from build123d import *

# Parameters (mm, degrees)
F1_DEPTH = 8.636


with BuildPart() as f1:
    # F0 (on Front) → F1 (new body)
    with BuildSketch(Plane.XZ):
        with BuildLine():
            Line((-67.888543, 14.229136), (-67.888543, 8.327846))
            Line((-67.888543, 8.327846), (-67.590117, 5.694489))
            Line((-67.590117, 5.694489), (-10.072526, 2.980128))
            Line((-10.072526, 2.980128), (-3.732844, -4.12088))
            Line((-3.732844, -4.12088), (2.804628, -4.12088))
            Line((2.804628, -4.12088), (4.660426, -5.51241))
            Line((4.660426, -5.51241), (20.36539, -5.51241))
            ThreePointArc((20.36539, -5.51241), (22.326214, -6.957719), (24.524612, -8.006907))
            ThreePointArc((24.524612, -8.006907), (28.372895, -8.935837), (32.329973, -9.052986))
            ThreePointArc((32.329973, -9.052986), (35.941526, -8.275719), (38.847856, -5.995215))
            ThreePointArc((38.847856, -5.995215), (42.405349, -6.590703), (44.239189, -9.696728))
            Line((44.239189, -9.696728), (45.717698, -10.69943))
            ThreePointArc((45.717698, -10.69943), (45.850918, -13.592314), (47.728516, -15.797116))
            ThreePointArc((47.728516, -15.797116), (48.186683, -17.808436), (48.07616, -19.868318))
            ThreePointArc((48.07616, -19.868318), (47.693475, -23.337022), (49.28254, -26.443986))
            ThreePointArc((49.28254, -26.443986), (49.565033, -26.802415), (49.898703, -27.113765))
            Line((49.898703, -27.113765), (63.92391, -23.246003))
            Line((63.92391, -23.246003), (63.666757, -17.629698))
            Line((63.666757, -17.629698), (63.305743, -9.745057))
            ThreePointArc((63.305743, -9.745057), (62.05497, -4.640389), (59.587408, 0))
            ThreePointArc((59.587408, 0), (55.333048, 5.257953), (53.080335, 11.635331))
            Line((53.080335, 11.635331), (51.798906, 15.11586))
            Line((51.798906, 15.11586), (46.942841, 15.11586))
            ThreePointArc((46.942841, 15.11586), (46.45979, 13.035678), (45.55238, 11.102519))
            ThreePointArc((45.55238, 11.102519), (43.355932, 7.020729), (39.016269, 5.392008))
            Line((39.016269, 5.392008), (23.084078, 5.392008))
            Line((23.084078, 5.392008), (23.084078, 6.470653))
            Line((23.084078, 6.470653), (15.109499, 6.470653))
            Line((15.109499, 6.470653), (13.445796, 6.470653))
            Line((13.445796, 6.470653), (13.445796, 11.590629))
            Line((13.445796, 11.590629), (13.445796, 18.615682))
            Line((13.445796, 18.615682), (7.789209, 18.615682))
            Line((7.789209, 18.615682), (-7.699287, 18.537793))
            Line((-7.699287, 18.537793), (-4.879672, 18.475959))
            Line((-4.879672, 18.475959), (-4.879672, 14.229136))
            Line((-4.879672, 14.229136), (-7.699287, 14.229136))
            Line((-7.699287, 14.229136), (-67.888543, 14.229136))
        make_face()
        with BuildLine():
            ThreePointArc((18.888429, -1.232992), (20.03881, 1.476523), (22.555076, 3.004023))
            Line((22.555076, 3.004023), (28.890261, 3.004023))
            Line((28.890261, 3.004023), (32.984652, 3.004023))
            ThreePointArc((32.984652, 3.004023), (33.457255, 2.948329), (33.923268, 2.851961))
            ThreePointArc((33.923268, 2.851961), (37.989765, -1.51717), (35.673525, -7.018146))
            ThreePointArc((35.673525, -7.018146), (28.392646, -7.940351), (21.466842, -5.51241))
            Line((21.466842, -5.51241), (18.888429, -1.232992))
        make_face(mode=Mode.SUBTRACT)
        Polygon((-67.26525, 18.70371), (-67.888543, 14.229136), (-7.699287, 14.229136), (-7.699287, 18.537793), (-66.731323, 18.629336), align=None)
        Polygon((-65.611368, 15.894235), (-65.609761, 16.930796), (-61.958702, 16.97587), (-61.958702, 15.888571), align=None, mode=Mode.SUBTRACT)
        Polygon((-66.731323, 21.379774), (-66.731323, 18.629336), (-7.699287, 18.537793), (7.789209, 18.615682), (13.445796, 18.615682), (13.445796, 20.43255), (13.445796, 23.939529), (11.8609, 24.011148), (10.443351, 22.458594), (3.288107, 22.458594), (2.613084, 23.025269), (-3.514589, 23.025269), (-3.514589, 19.527677), (-59.21186, 19.614049), (-60.399957, 21.379774), align=None)
        Polygon((-66.20314, 22.302656), (-66.731323, 21.379774), (-60.399957, 21.379774), (-14.40332, 21.379774), (-13.479427, 23.025269), (-3.514589, 23.025269), (2.613084, 23.025269), (2.580326, 23.198023), (-17.181331, 23.198023), (-17.794525, 22.302656), align=None)
        with BuildLine():
            Line((-66.731323, 23.473777), (-66.20314, 22.302656))
            Line((-66.20314, 22.302656), (-17.794525, 22.302656))
            Line((-17.794525, 22.302656), (-17.181331, 23.198023))
            Line((-17.181331, 23.198023), (2.580326, 23.198023))
            Line((2.580326, 23.198023), (2.613084, 23.025269))
            Line((2.613084, 23.025269), (3.288107, 22.458594))
            Line((3.288107, 22.458594), (10.443351, 22.458594))
            Line((10.443351, 22.458594), (11.8609, 24.011148))
            Line((11.8609, 24.011148), (13.445796, 23.939529))
            Line((13.445796, 23.939529), (34.916848, 23.939529))
            Line((34.916848, 23.939529), (34.916848, 22.35744))
            Line((34.916848, 22.35744), (36.640268, 22.35744))
            Line((36.640268, 22.35744), (36.640268, 21.295426))
            Line((36.640268, 21.295426), (37.662946, 20.430082))
            Line((37.662946, 20.430082), (37.662946, 18.97577))
            Line((37.662946, 18.97577), (42.068332, 13.861337))
            Line((42.068332, 13.861337), (42.068332, 9.9928))
            Line((42.068332, 9.9928), (37.926942, 9.9928))
            Line((37.926942, 9.9928), (36.640268, 8.652356))
            Line((36.640268, 8.652356), (36.640268, 7.140663))
            Line((36.640268, 7.140663), (39.016269, 7.140663))
            ThreePointArc((39.016269, 7.140663), (40.885778, 7.338312), (42.642005, 8.008977))
            ThreePointArc((42.642005, 8.008977), (44.260743, 9.401881), (45.55238, 11.102519))
            ThreePointArc((45.55238, 11.102519), (46.45979, 13.035678), (46.942841, 15.11586))
            Line((46.942841, 15.11586), (51.798906, 15.11586))
            Line((51.798906, 15.11586), (51.798906, 16.040822))
            Line((51.798906, 16.040822), (45.381963, 19.682869))
            Line((45.381963, 19.682869), (42.202402, 18.006373))
            Line((42.202402, 18.006373), (40.930577, 18.006373))
            Line((40.930577, 18.006373), (38.329113, 19.682869))
            Line((38.329113, 19.682869), (38.329113, 25.174845))
            Line((38.329113, 25.174845), (38.329113, 28.956141))
            Line((38.329113, 28.956141), (16.867928, 28.956141))
            Line((16.867928, 28.956141), (15.879637, 29.998008))
            Line((15.879637, 29.998008), (15.187833, 29.998008))
            Line((15.187833, 29.998008), (11.387558, 29.998008))
            Line((11.387558, 29.998008), (5.248655, 27.211197))
            Line((5.248655, 27.211197), (-54.899268, 27.211197))
            Line((-54.899268, 27.211197), (-61.934408, 27.211197))
            Line((-61.934408, 27.211197), (-65.839738, 27.211197))
            Line((-65.839738, 27.211197), (-65.839738, 25.936976))
            Line((-65.839738, 25.936976), (-66.731323, 24.311243))
            Line((-66.731323, 24.311243), (-66.731323, 23.473777))
        make_face()
        with BuildLine():
            ThreePointArc((-63.038021, 24.306566), (-63.715772, 25.131149), (-63.090824, 25.996437))
            ThreePointArc((-63.090824, 25.996437), (-62.267006, 25.176418), (-63.038021, 24.306566))
        make_face(mode=Mode.SUBTRACT)
        with BuildLine():
            ThreePointArc((-54.377425, 24.306566), (-55.235893, 25.101148), (-54.483041, 25.996437))
            ThreePointArc((-54.483041, 25.996437), (-53.73549, 25.194922), (-54.377425, 24.306566))
        make_face(mode=Mode.SUBTRACT)
        Polygon((-50.948696, 24.560757), (-51.789809, 25.860662), (-22.338423, 26.090056), (-21.319148, 24.51481), align=None, mode=Mode.SUBTRACT)
        Polygon((-2.707183, 24.560757), (-19.452998, 24.560757), (-20.294111, 26.090056), (-3.548297, 26.090056), align=None, mode=Mode.SUBTRACT)
        Polygon((-61.934408, 29.162308), (-61.934408, 27.211197), (-54.899268, 27.211197), (-56.723192, 29.162308), align=None)
        Polygon((63.92391, -23.246003), (49.898703, -27.113765), (47.567636, -29.108122), (48.197687, -29.844546), (47.567636, -30.38359), (60.629882, -27.680274), (61.969539, -25.573865), (66.964559, -24.576284), (66.767075, -23.464401), (65.788557, -23.509205), (65.665543, -20.822546), (65.180847, -20.337525), (65.090388, -18.361883), (63.666757, -17.629698), align=None)
        Polygon((42.202402, 18.006373), (45.381963, 19.682869), (44.331331, 20.500985), (40.165214, 23.745094), (38.329113, 25.174845), (38.329113, 19.682869), (40.930577, 18.006373), align=None)
        with BuildLine():
            Line((40.165214, 23.745094), (44.331331, 20.500985))
            Line((44.331331, 20.500985), (44.331331, 22.302926))
            ThreePointArc((44.331331, 22.302926), (45.705089, 24.725057), (48.342105, 25.619529))
            ThreePointArc((48.342105, 25.619529), (44.854467, 25.661592), (41.94029, 23.745094))
            Line((41.94029, 23.745094), (40.165214, 23.745094))
        make_face()
        Polygon((60.629882, -27.680274), (47.567636, -30.38359), (47.567636, -30.86937), (51.254567, -32.621317), (65.507576, -30.38359), (67.471333, -27.113765), (66.964559, -24.576284), (61.969539, -25.573865), align=None)
        with BuildLine():
            ThreePointArc((64.190447, -28.582929), (62.846638, -27.292852), (64.190447, -26.002776))
            ThreePointArc((64.190447, -26.002776), (65.423903, -27.292852), (64.190447, -28.582929))
        make_face(mode=Mode.SUBTRACT)
    extrude(amount=F1_DEPTH)


solid = f1.part
Geometry check sheet. Reference: the model listing, model coordinates, mm. A direction names the side the tool comes from. Give positions to 0.01 mm unless a question says otherwise; leave off trailing zeros. Answer in a Markdown table with one row per item. Add a question column.
1) Draft check along X on faces 6 (the face through (66.476, -4.258, -28.772)), 7 (the face through (-67.889, -4, 11)), 8 (the face through (-1, -4, -4.121)), 9 (the face through (-24, -4, 27.211)). Enter one of: pulls with the +X half, pulls with the -X half, needs draft (parallel to the pull), parting line crosses it, or undercut.
2) Gauge pin test, flat ends, axial feed: P1, Ø4.5, axis at x = 34.5, y = -2.5, coming from the +Z side; P2, Ø2, axis at y = -2.5, z = 20, coming from the -X side; P3, Ø4.5, axis at x = 23, y = -3.5, coming from the -Z side. Record the tip position at first contact, or that the pin passes through.
3) Set-up check for faces 1 (the face through (-59, -4, 29.162)), 2 (the face through (12, -4, -5.512)), 3 (the face through (48.635, -4.258, 17.836)), 4 (the face through (13.446, -4, 15)), 5 (the face through (38.329, -4, 27)): record each of +Z, -Z, +X, -X, +Y, -Y from which the full face is reachable in a straight line by a thin tool's end or side.
4) Material ranges on probe 1 along X at (y, z) = (-8, 25); probe 2 along Z at (x, y) = (-37, -3); probe 3 along Z at (x, y) = (45, -0.25), recorded low to high. Write a range as from..to.
5) Cross-section at A-A on y = -4.25. State how many separate pieces and enclosed holes the cut face has, and give its area (3 significant figures).
Outcome:
| question | item | result |
|---|---|---|
| 1 | face 6 | pulls with the +X half |
| 1 | face 7 | pulls with the -X half |
| 1 | face 8 | needs draft |
| 1 | face 9 | undercut |
| 2 | P1 | stops at z = 28.96 |
| 2 | P2 | stops at x = -66.73 |
| 2 | P3 | stops at z = -8.25 |
| 3 | face 1 | +Z, -X, +Y, -Y |
| 3 | face 2 | -Z, -X, +Y, -Y |
| 3 | face 3 | +X, +Y, -Y |
| 3 | face 4 | +Y, -Y |
| 3 | face 5 | +Z, +Y, -Y |
| 4 | probe 1 | x = -66.35..-63.7, -62.28..-55.22, -53.75..-51.23, -21.63..-19.69, -2.95..38.55, 43.38..46.08 |
| 4 | probe 2 | z = 4.25..19.58, 21.38..24.54, 25.98..27.21 |
| 4 | probe 3 | z = -10.21..9.21, 10.28..19.98, 23.96..25.7 |
| 5 | separate pieces | 1 |
| 5 | enclosed holes | 10 |
| 5 | area | 3,040 mm^2 |
